Read the model definition and answer for the solid it produces. Units are mm, in the model's axes. Round coordinates to 2 decimals unless told otherwise and drop trailing zeros. Loops run counter-clockwise (first coordinate to the right, second up) from the corner with the lowest first, then second, coordinate; pieces in that order, holes last. Notation, with made-up numbers: (-31, 43.25) - (28, 43.25) arc R15 cw to (28, 67.25) - close; hole circle Ø3 at (-23.75, -7.5). An arc over 180 degrees is marked (long way). Use CSV: the item, a comma, the result in double quotes. Start each with the question number.
1. Find section B-B (y = 0). Give the vertices of the cut face in (x, z).
2. Find section C-C (z = 1). Give the vertices of the cut face in (x, y) (1 decimal), and give its area (3 significant figures).
3. Find section A-A (x = 0). Give the vertices of the cut face in (y, z).
4. Consider line 1 along Y through (x, z) = (0, 2.1); line 2 along X through (y, z) = (0, 1.4); line 3 along X through (y, z) = (-4, 1.4). Determine where each line is inside the solid, lowest interval first.
5. Given pin 1 Ø5.5 at (x, y) = (-15.16, -8.75) entering from +Z; pin 2 Ø4 at (x, y) = (0, 15.155) entering from +Z, each flat-ended and moving along its own axis, determine where each tip first touches the part or whether it passes through.
6. Find section D-D (x = 9). Give the vertices of the cut face in (y, z), and give its area (3 significant figures).
Autodesk Inventor part; units mm, degrees
ref_plane "YZ Plane" through (0, 0, 0) normal (1, 0, 0) x (0, 1, 0)
ref_plane "XZ Plane" through (0, 0, 0) normal (0, 1, 0) x (-1, 0, 0)
ref_plane "XY Plane" through (0, 0, 0) normal (0, 0, 1) x (1, 0, 0)
sketch "Sketch1" plane through (0, 0, 0) normal (0, 0, 1) x (1, 0, 0)
  line L0 (-20, -20) -> (20, -20)
  line L1 (20, -20) -> (20, 20)
  line L2 (20, 20) -> (-20, 20)
  line L3 (-20, 20) -> (-20, -20)
  line L4 (-20, -20) -> (20, 20) construction
  line L5 (20, -20) -> (-20, 20) construction
  circle A0 centre (0, 0) radius 11
  line L6 (0, 0) -> (0, 15.155)
  line L7 (0, 0) -> (15.155, -8.7497)
  line L8 (0, 0) -> (-15.155, -8.7497)
  circle A1 centre (0, 15.155) radius 2.3575
  circle A2 centre (15.155, -8.7497) radius 2.3575
  circle A3 centre (-15.155, -8.7497) radius 2.3575
  dimension "d0" = 40
  dimension "d1" = 40
  dimension "d2" = 22
  dimension "d3" = 15.155
  dimension "d4" = 15.155
  dimension "d5" = 120
  dimension "d6" = 15.155
  dimension "d7" = 120
  dimension "d8" = 4.715
  dimension "d9" = 4.715
  dimension "d10" = 4.715
extrude "Extrusion1" add sketch "Sketch1" along normal blind 3
equation "\"d1\" = d0"
equation "\"d4\" = d3"
equation "\"d6\" = d3"
equation "\"d7\" = d5"
equation "\"d9\" = d8"
equation "\"d10\" = d8"
properties part number "mount_v01"
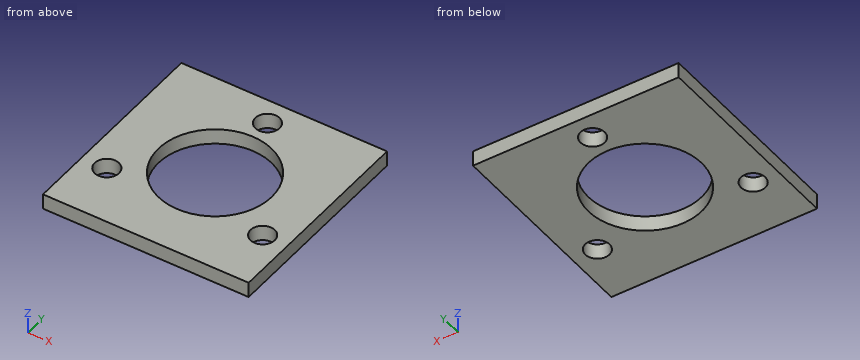
Filled sheet:
1,outline,"(-20, 0) - (-11, 0) - (-11, 3) - (-20, 3) - close; (11, 0) - (20, 0) - (20, 3) - (11, 3) - close"
2,outline,"(-20, -20) - (20, -20) - (20, 20) - (-20, 20) - close; hole circle Ø4.7 at (-15.2, -8.7); hole circle Ø22 at (0, 0); hole circle Ø4.7 at (0, 15.2); hole circle Ø4.7 at (15.2, -8.7)"
2,area,"1,170 mm²"
3,outline,"(-20, 0) - (-11, 0) - (-11, 3) - (-20, 3) - close; (11, 0) - (12.8, 0) - (12.8, 3) - (11, 3) - close; (17.51, 0) - (20, 0) - (20, 3) - (17.51, 3) - close"
4,line 1,"y = -20 to -11, 11 to 12.8, 17.51 to 20"
4,line 2,"x = -20 to -11, 11 to 20"
4,line 3,"x = -20 to -10.25, 10.25 to 20"
5,pin 1,"stops at z = 3"
5,pin 2,"passes through"
6,outline,"(-20, 0) - (-6.32, 0) - (-6.32, 3) - (-20, 3) - close; (6.32, 0) - (20, 0) - (20, 3) - (6.32, 3) - close"
6,area,"82.1 mm²"
